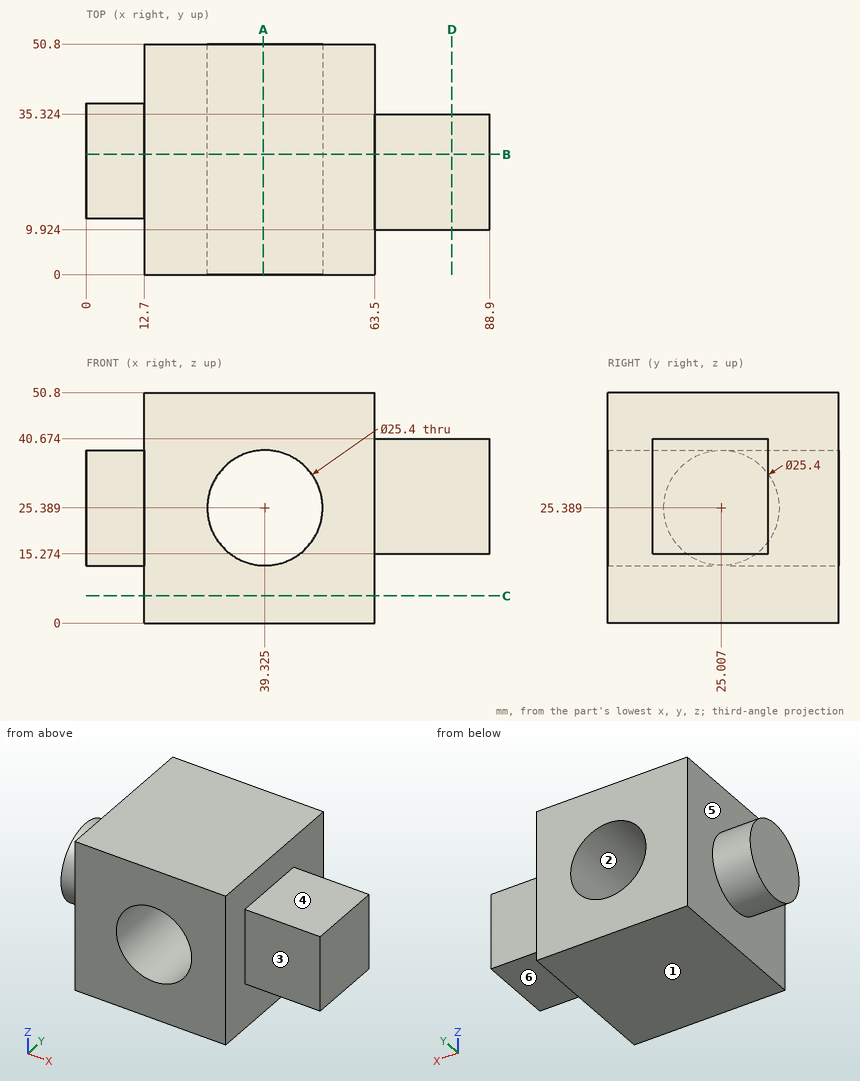
Part print with two shaded views. Sizes in mm from the minimum x, y, z corner. A direction names the side the tool comes from. Coordinates: 2 decimals unless noted, no trailing zeros. Write each loop counter-clockwise with the first axis right and the second up, starting at its lowest first coordinate (ties: lowest second). Pieces come first, ordered by that corner, then holes. Notation, with made-up numbers: (11, 2) -> (55, 2) arc R32 cw to (55, 34) -> close; hole circle Ø1 at (-2, -24). An arc over 180 degrees is marked (long way). Return JSON: item names as keys, results as strings. Group by question number.
Q1. Cut at C-C, the plane z = 6. Give the cut face in (x, y).
Q2. Cut at B-B, the plane y = 26.5. Give the cut face in (x, z) (1 decimal).
Q3. Cut at A-A, the plane x = 39. Give the cut face in (y, z) (1 decimal).
Q4. Pull direction Z, two halves, no side cores. Call the marked faces 1, 2 and 3: released by +Z, released by -Z, zero draft, split by the parting line, or undercut.
Q5. Flat gauge pins, fed straight in: pin 1 (20.5 mm diameter, centred on x = 73.5, z = 22.5, fed in from -Y); pin 2 (3 mm diameter, centred on y = 10, z = 43.5, fed in from +X); pin 3 (12.5 mm diameter, centred on x = 73.5, z = 25, fed in from +Y); pin 4 (20.5 mm diameter, centred on x = 79.5, y = 22.5, fed in from +Z). Where does each tip first touch, or does it go through?
Q6. Drill centre lines: line 1 (Z direction, x = 39, y = 19.5) (1 decimal); line 2 (X direction, y = 44, z = 25.5) (1 decimal); line 3 (Z direction, x = 73, y = 34). Where is each one in solid material? Low to high.
Q7. Which spindle directions (+Z, -Z, +X, -X, +Y, -Y) get a long thin tool onto all of the face, cutting with end or side? Do the marked faces 4, 5 and 6. Say none if no direction does.
Q8. Cut at D-D, the plane x = 80.5. Give the cut face in (y, z), then the cut area to 3 significant figures.
Returned:
{
 "1": {"outline": "(12.7, 0) -> (63.5, 0) -> (63.5, 50.8) -> (12.7, 50.8) -> close"},
 "2": {"outline": "(0, 12.8) -> (12.7, 12.8) -> (12.7, 0) -> (63.5, 0) -> (63.5, 15.3) -> (88.9, 15.3) -> (88.9, 40.7) -> (63.5, 40.7) -> (63.5, 50.8) -> (12.7, 50.8) -> (12.7, 38) -> (0, 38) -> close; hole circle Ø25.4 at (39.3, 25.4)"},
 "3": {"outline": "(0, 0) -> (50.8, 0) -> (50.8, 12.7) -> (0, 12.7) -> close; (0, 38.1) -> (50.8, 38.1) -> (50.8, 50.8) -> (0, 50.8) -> close"},
 "4": {"face 1": "released by -Z", "face 2": "undercut", "face 3": "zero draft"},
 "5": {"pin 1": "stops at y = 0", "pin 2": "stops at x = 63.5", "pin 3": "stops at y = 35.32", "pin 4": "stops at z = 40.67"},
 "6": {"line 1": "z = 0 to 12.7, 38.1 to 50.8", "line 2": "x = 12.7 to 26.6, 52 to 63.5", "line 3": "z = 15.27 to 40.67"},
 "7": {"face 4": "+Z, +X, +Y, -Y", "face 5": "-X", "face 6": "-Z, +X, +Y, -Y"},
 "8": {"outline": "(9.92, 15.27) -> (35.32, 15.27) -> (35.32, 40.67) -> (9.92, 40.67) -> close", "area": "645 mm2"}
}
